Model file for the job. Use its own axes, mm. Coordinates: 2 decimals unless noted, no trailing zeros. Loops run counter-clockwise (first coordinate to the right, second up) from the corner with the lowest first, then second, coordinate; pieces in that order, holes last. Notation, with made-up numbers: M -14,-7.5 L 13,-7.5 A26 cw 13,28.5 Z; hole C 0.5,0 d10. An arc over 180 degrees is marked long. Write item = value, one per line. Start each with the question number.
from build123d import *

# Parameters (mm, degrees)
BOSS_EXTRUDE1_DEPTH = 2
SKETCH2_R           = 1.6
SKETCH2_R_2         = 7.5
CUT_EXTRUDE1_DEPTH  = 82.192672083


with BuildPart() as part:
    # Sketch1 → Boss-Extrude1 (new body)
    with BuildSketch(Plane.XY):
        Polygon((76, 28.5), (-76, 28.5), (-76, 5), (-74, 5), (-74, -5), (-76, -5), (-76, -28.5), (76, -28.5), (76, -5), (74, -5), (74, 5), (76, 5), align=None)
    extrude(amount=BOSS_EXTRUDE1_DEPTH)

    # Sketch2 → Cut-Extrude1 (cut, through all)
    with BuildSketch(Plane.XY.offset(2)):
        with Locations((-72.5, 24.05)):
            Circle(SKETCH2_R)
        with Locations((72.5, 24.05)):
            Circle(SKETCH2_R)
        with Locations((66, -24.05)):
            Circle(SKETCH2_R)
        with Locations((-66, -24.05)):
            Circle(SKETCH2_R)
        with Locations((-56, 0)):
            Circle(SKETCH2_R_2)
    extrude(amount=-CUT_EXTRUDE1_DEPTH, mode=Mode.SUBTRACT)


solid = part.part
Item 1: Cut at A-A (y = 0). Give the cut face in (x, z), plus the area to 3 significant figures.
Item 2: Probe L1, parallel to Y at x = 66, z = 1.25; L2, parallel to Y at x = -72.5, z = 1.1; L3, parallel to X at y = 1.5, z = 0.1. List the from-to ranges inside material, lowest first.
Item 3: Cut at C-C (z = 1.3). Give the cut face in (x, y).
Item 4: Cut at D-D (y = -24.05). Give the cut face in (x, z).
Item 5: Cut at B-B (x = -56). Give the cut face in (y, z).
Item 6: Pin check, flat tips, straight feed: pin 1 Ø1 at (y, z) = (-1.5, 1.5) entering from -X; pin 2 Ø5 at (x, y) = (72.5, 24.05) entering from -Z; pin 3 Ø2.5 at (x, y) = (66, -24.05) entering from +Z; pin 4 Ø1 at (y, z) = (-2, 0.5) entering from +X. Stop position of each tip, or through.
Item 7: Pull direction X, two halves, no side cores. Call faces 1 (the cylindrical face through (-64.474, -23.569, 1.014)), 2 (the flat face through (-1, 0, 2)): +X half, -X half, draft (parallel to the pull), parting line (faces both ways), or undercut.
Reported:
q1.outline = M -74,0 L -63.5,0 L -63.5,2 L -74,2 Z; M -48.5,0 L 74,0 L 74,2 L -48.5,2 Z
q1.area = 266 mm^2
q2.L1 = -28.5 to -25.65, -22.45 to 28.5
q2.L2 = -28.5 to 22.45, 25.65 to 28.5
q2.L3 = -74 to -63.35, -48.65 to 74
q3.outline = M -76,-28.5 L 76,-28.5 L 76,-5 L 74,-5 L 74,5 L 76,5 L 76,28.5 L -76,28.5 L -76,5 L -74,5 L -74,-5 L -76,-5 Z; hole C -72.5,24.05 d3.2; hole C -66,-24.05 d3.2; hole C -56,0 d15; hole C 66,-24.05 d3.2; hole C 72.5,24.05 d3.2
q4.outline = M -76,0 L -67.6,0 L -67.6,2 L -76,2 Z; M -64.4,0 L 64.4,0 L 64.4,2 L -64.4,2 Z; M 67.6,0 L 76,0 L 76,2 L 67.6,2 Z
q5.outline = M -28.5,0 L -7.5,0 L -7.5,2 L -28.5,2 Z; M 7.5,0 L 28.5,0 L 28.5,2 L 7.5,2 Z
q6.pin_1 = -74
q6.pin_2 = 0
q6.pin_3 = through
q6.pin_4 = 74
q7.face_1 = undercut
q7.face_2 = draft
